```python
from build123d import *

# Parameters (mm, degrees)
F0_W      = 50
F0_H      = 40
F1_DEPTH  = 40
F2_W      = 10
F2_H      = 20
F3_DEPTH  = 50.001
F4_W      = 30
F4_H      = 10
F5_DEPTH  = 20.001
F6_W      = 10
F6_H      = 20
F7_DEPTH  = 20
F9_DEPTH  = 30.001
F10_DEPTH = 30.001


with BuildPart() as f1:
    # F0 (on Front) → F1 (new body)
    with BuildSketch(Plane.XZ):
        with Locations((25, 20)):
            Rectangle(F0_W, F0_H)
    extrude(amount=F1_DEPTH)

    # F2 (on face) → F3 (cut, through all)
    with BuildSketch(Plane(origin=(0, 0, 0), x_dir=(0, -1, 0), z_dir=(-1, 0, 0))):
        with Locations((5, 30)):
            Rectangle(F2_W, F2_H)
        with Locations((35, 30)):
            Rectangle(F2_W, F2_H)
    extrude(amount=-F3_DEPTH, mode=Mode.SUBTRACT)

    # F4 (on face) → F5 (cut, through all)
    with BuildSketch(Plane.XY.offset(20)):
        with Locations((15, -5)):
            Rectangle(F4_W, F4_H)
        with Locations((15, -35)):
            Rectangle(F4_W, F4_H)
    extrude(amount=-F5_DEPTH, mode=Mode.SUBTRACT)

    # F6 (on face) → F7 (cut, through all)
    with BuildSketch(Plane.XY.offset(40)):
        with Locations((45, -20)):
            Rectangle(F6_W, F6_H)
    extrude(amount=-F7_DEPTH, mode=Mode.SUBTRACT)

    # F8 (on face) → F9 (cut, through all)
    with BuildSketch(Plane.XZ.offset(30)):
        Polygon((10, 40), (0, 40), (0, 20), align=None)
    extrude(amount=-F9_DEPTH, mode=Mode.SUBTRACT)

    # F8 (on face) → F10 (cut, through all)
    with BuildSketch(Plane.XZ.offset(30)):
        Polygon((10, 0), (0, 20), (0, 0), align=None)
    extrude(amount=-F10_DEPTH, mode=Mode.SUBTRACT)


solid = f1.part
```
CAD build for the part. Positions are in the model's coordinates, mm. A direction names the side the tool comes from. Give positions to 0.01 mm unless a question says otherwise; leave off trailing zeros. Order: outer loops, then holes, each group sorted by start corner. A loop starts at its lowest first (then second) coordinate and runs counter-clockwise, first axis right, second up.
(1) Tool access for faces 1 (the flat face through (40, -20, 30)), 2 (the flat face through (30, -5, 10)), 3 (the flat face through (30, -35, 10)): list every direction of +Z, -Z, +X, -X, +Y, -Y with a clear straight run to the whole face (end or side of a thin tool).
(2) Drill centre lines: L1, parallel to Z at x = 31, y = -5; L2, parallel to Y at x = 20.5, z = 20.5; L3, parallel to X at y = -35, z = 9. Where is each one in solid material? Low to high.
(3) Saw through at A-A, the plane z = 19. Give the cut face in (x, y).
(4) Flat gauge pins, fed straight in: pin 1 (12 mm diameter, centred on x = 12, z = 20, fed in from +Y); pin 2 (5 mm diameter, centred on y = -37.5, z = 9.5, fed in from -X); pin 3 (1.5 mm diameter, centred on y = -11, z = 13.5, fed in from -X) (3 decimals). Where does each tip first touch, or does it go through?
(5) Saw through at C-C, the plane z = 6.5. Give the cut face in (x, y).
(6) Saw through at D-D, the plane x = 5. Give the cut face in (y, z).
(7) Saw through at B-B, the plane y = -26. Give the cut face in (x, z).
Results found:
1. face 1: +Z, +X, +Y, -Y
1. face 2: +Z, -Z, -X, +Y
1. face 3: +Z, -Z, -X, -Y
2. L1: z = 0 to 20
2. L2: y = -30 to -10
2. L3: x = 30 to 50
3. outline: (0.5, -30) - (30, -30) - (30, -40) - (50, -40) - (50, 0) - (30, 0) - (30, -10) - (0.5, -10) - close
4. pin 1: stops at y = -10
4. pin 2: stops at x = 30
4. pin 3: stops at x = 2.875
5. outline: (6.75, -30) - (30, -30) - (30, -40) - (50, -40) - (50, 0) - (30, 0) - (30, -10) - (6.75, -10) - close
6. outline: (-30, 10) - (-10, 10) - (-10, 30) - (-30, 30) - close
7. outline: (0, 20) - (10, 0) - (50, 0) - (50, 20) - (40, 20) - (40, 40) - (10, 40) - close
